from build123d import *

# Parameters (mm, degrees)
SKETCH1_R           = 3.429
SKETCH1_R_2         = 2.54
BOSS_EXTRUDE1_DEPTH = 3.2004
SKETCH5_R           = 2.159
SKETCH5_W           = 40.894
SKETCH5_H           = 20.32
CUT_EXTRUDE3_DEPTH  = 4.2004
CUT_EXTRUDE4_DEPTH  = 3.2004
CUT_EXTRUDE5_DEPTH  = 3.2004
SKETCH9_R           = 2.159
SKETCH9_W           = 2.54
SKETCH9_H           = 3.81
BOSS_EXTRUDE2_DEPTH = 3.2004
FILLET1_R           = 2.54


with BuildPart() as part:
    # Sketch1 → Boss-Extrude1 (new body)
    with BuildSketch(Plane.XY):
        with BuildLine():
            Line((120.015, 37.81552), (0, 37.81552))
            ThreePointArc((0, 37.81552), (-18.90776, 18.90776), (0, 0))
            Line((0, 0), (120.015, 0))
            ThreePointArc((120.015, 0), (138.92276, 18.90776), (120.015, 37.81552))
        make_face()
        with Locations((120.015, 18.90776)):
            Circle(SKETCH1_R, mode=Mode.SUBTRACT)
        with Locations((0, 18.90776)):
            Circle(SKETCH1_R_2, mode=Mode.SUBTRACT)
    extrude(amount=BOSS_EXTRUDE1_DEPTH)

    # Sketch5 → Cut-Extrude3 (cut, through all)
    with BuildSketch(Plane(origin=(0, 0, 0), x_dir=(-1, 0, 0), z_dir=(0, 0, -1))):
        with Locations((-79.746999972, 23.90776)):
            Circle(SKETCH5_R)
        with Locations((-29.246999972, 13.90776)):
            Circle(SKETCH5_R)
        with Locations((-29.246999972, 23.90776)):
            Circle(SKETCH5_R)
        with Locations((-79.746999972, 13.90776)):
            Circle(SKETCH5_R)
        with Locations((-92.322240346, 23.90776)):
            Circle(SKETCH5_R)
        with Locations((-92.322240346, 13.90776)):
            Circle(SKETCH5_R)
        with Locations((-54.496999972, 18.90776)):
            Rectangle(SKETCH5_W, SKETCH5_H)
    extrude(amount=-CUT_EXTRUDE3_DEPTH, mode=Mode.SUBTRACT)

    # Sketch6 → Cut-Extrude4 (cut)
    with BuildSketch(Plane.XY.offset(3.2004)):
        with BuildLine():
            Line((8.649999972, 20.49526), (25.159999972, 20.49526))
            ThreePointArc((25.159999972, 20.49526), (26.747499972, 18.90776), (25.159999972, 17.32026))
            Line((25.159999972, 17.32026), (8.649999972, 17.32026))
            ThreePointArc((8.649999972, 17.32026), (7.062499972, 18.90776), (8.649999972, 20.49526))
        make_face()
    extrude(amount=-CUT_EXTRUDE4_DEPTH, mode=Mode.SUBTRACT)

    # Sketch8 → Cut-Extrude5 (cut)
    with BuildSketch(Plane.XY.offset(3.2004)):
        Polygon((34.049999972, 15.79626), (34.049999972, 22.01926), (23.264769203, 20.49526), (23.264769203, 17.32026), align=None)
    extrude(amount=-CUT_EXTRUDE5_DEPTH, mode=Mode.SUBTRACT)

    # Sketch9 → Boss-Extrude2 (add)
    with BuildSketch(Plane(origin=(0, 0, 0), x_dir=(-1, 0, 0), z_dir=(0, 0, -1))):
        with BuildLine():
            Line((-40.703500071, 37.81552), (-15.303500071, 37.81552))
            Line((-15.303500071, 37.81552), (-20.042454023, 71.094701578))
            ThreePointArc((-20.042454023, 71.094701578), (-21.381188491, 73.552326238), (-24.003000071, 74.531219996))
            Line((-24.003000071, 74.531219996), (-32.004000071, 74.531219996))
            ThreePointArc((-32.004000071, 74.531219996), (-34.62581165, 73.552326238), (-35.964546118, 71.094701578))
            Line((-35.964546118, 71.094701578), (-40.703500071, 37.81552))
        make_face()
        with Locations((-32.004000071, 70.53072)):
            Circle(SKETCH9_R, mode=Mode.SUBTRACT)
        with Locations((-24.003000071, 70.53072)):
            Circle(SKETCH9_R, mode=Mode.SUBTRACT)
        with Locations((-31.178500071, 55.533488225)):
            Rectangle(SKETCH9_W, SKETCH9_H, mode=Mode.SUBTRACT)
        with Locations((-24.828500071, 55.533488225)):
            Rectangle(SKETCH9_W, SKETCH9_H, mode=Mode.SUBTRACT)
    extrude(amount=-BOSS_EXTRUDE2_DEPTH)

    # Fillet1
    fillet1_edges = [part.edges().sort_by_distance(p)[0] for p in [
        (34.049999972, 22.01926, 1.6002),
        (23.264769203, 20.49526, 1.6002),
        (23.264769203, 17.32026, 1.6002),
        (34.049999972, 15.79626, 1.6002),
    ]]
    fillet(fillet1_edges, radius=FILLET1_R)


solid = part.part
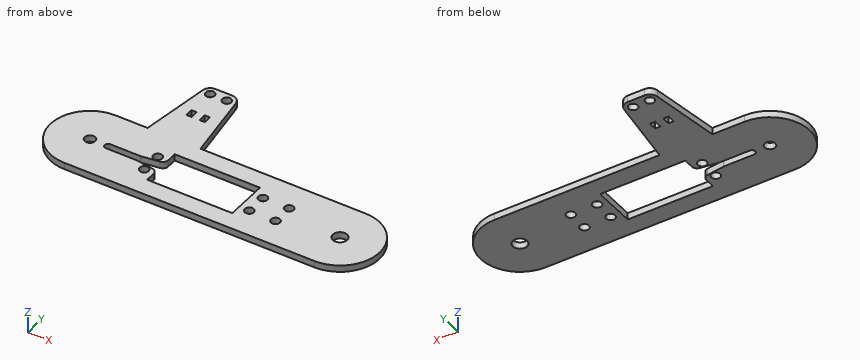
Check sheet for the modelled part. Datum: model origin and axes. Units: mm. Round coordinates to 2 decimals unless told otherwise and drop trailing zeros. Write each loop counter-clockwise with the first axis right and the second up, starting at its lowest first coordinate (ties: lowest second). Pieces come first, ordered by that corner, then holes. Notation, with made-up numbers: (17.5, 4.25) - (22.5, 4.25) arc R5 ccw to (22.5, 8.25) - close; hole circle Ø2 at (47.5, 86.5). An arc over 180 degrees is marked (long way). Return JSON: item names as keys, results as strings.
Q1. Scan lines: L1, parallel to X at y = 19, z = 2.65; L2, parallel to Y at x = 55, z = 2; L3, parallel to Y at x = 33.5, z = 0.5. Record each from-to range of solid material in increasing order. Write a range as from..to.
Returned:
{"L1": "x = -18.91..-2.54, 2.54..7.07, 74.94..116.59, 123.44..138.92", "L2": "y = 0..8.75, 29.07..37.82", "L3": "y = 0..15.17, 22.65..68.97, 72.09..74.24"}
Q2. Cross-section at C-C (x = 108.5). Record the boundary of the cut face in (y, z).
Returned:
{"outline": "(0, 0) - (37.82, 0) - (37.82, 3.2) - (0, 3.2) - close"}
Q3. Cross-section at D-D (z = 2.3). Give the number of separate pieces and of enclosed holes in the cut face, then the cut area to 3 significant figures.
Returned:
{"separate pieces": "1", "enclosed holes": "13", "area": "5,270 mm²"}
Q4. Cross-section at B-B (y = 27.5). Record the boundary of the cut face in (x, z), then the cut area to 3 significant figures.
Returned:
{"outline": "(-16.84, 0) - (34.05, 0) - (34.05, 3.2) - (-16.84, 3.2) - close; (74.94, 0) - (136.86, 0) - (136.86, 3.2) - (74.94, 3.2) - close", "area": "361 mm²"}
Q5. Depth check by flat-ended pin: P1, Ø2.5, axis at x = 79.75, y = 23.91, coming from the -Z side; P2, Ø1, axis at y = 55, z = 1, coming from the -X side; P3, Ø1.6, axis at x = 91.5, z = 1, coming from the +Y side; P4, Ø1, axis at y = 56, z = 1, coming from the -X side. Enter the tip coordinate at first touch or a pass-through.
Returned:
{"P1": "passes through", "P2": "stops at x = 17.68", "P3": "stops at y = 37.82", "P4": "stops at x = 17.82"}
Q6. Cross-section at A-A (x = 48). Record the boundary of the cut face in (y, z), then the cut area to 3 significant figures.
Returned:
{"outline": "(0, 0) - (8.75, 0) - (8.75, 3.2) - (0, 3.2) - close; (29.07, 0) - (37.82, 0) - (37.82, 3.2) - (29.07, 3.2) - close", "area": "56.0 mm²"}
